Design review of the part built by this model. Coordinates are the model's own, in mm. Face numbers are marked on the shaded views. A direction names the side the tool comes from. Give positions to 0.01 mm unless a question says otherwise; leave off trailing zeros. Order: outer loops, then holes, each group sorted by start corner. A loop starts at its lowest first (then second) coordinate and runs counter-clockwise, first axis right, second up. Notation, with made-up numbers: M 76,-25 L 122,-25 A14 ccw 122,-20 Z; hole C -17.75,-0.75 d1. An arc over 180 degrees is marked long. Answer as a JSON object with one key per item and string values.
from build123d import *

# Parameters (mm, degrees)
F0_W     = 200
F0_H     = 164
F0_R     = 67
F0_H_2   = 12
F0_R_2   = 53
F1_DEPTH = 12
F2_W     = 12
F2_H     = 69
F2_H_2   = 12
F2_H_3   = 152
F2_W_2   = 6
F3_DEPTH = 276
F4_W     = 200
F4_H     = 257
F5_DEPTH = 12


with BuildPart() as f1:
    # F0 (on Front) → F1 (new body)
    with BuildSketch(Plane.XZ):
        with Locations((0, -46.5)):
            Rectangle(F0_W, F0_H)
        with Locations((0, -40.5)):
            Circle(F0_R, mode=Mode.SUBTRACT)
        Polygon((100, 128.5), (-100, 128.5), (-100, 47.5), (100, 47.5), (100, 67.5), (30, 67.5), (30, 108.5), (100, 108.5), align=None)
        with Locations((0, 41.5)):
            Rectangle(F0_W, F0_H_2)
        with Locations((0, -40.5)):
            Circle(F0_R)
        with Locations((0, -40.5)):
            Circle(F0_R_2, mode=Mode.SUBTRACT)
    extrude(amount=F1_DEPTH)

    # F2 (on face) → F3 (join)
    with BuildSketch(Plane(origin=(0, 0, 0), x_dir=(-1, 0, 0), z_dir=(0, 1, 0))):
        Polygon((100, 128.5), (-100, 128.5), (-100, 116.5), (88, 116.5), (100, 116.5), align=None)
        with Locations((94, 82)):
            Rectangle(F2_W, F2_H)
        with Locations((94, 41.5)):
            Rectangle(F2_W, F2_H_2)
        Polygon((88, 35.5), (88, 47.5), (-100, 47.5), (-100, 35.5), (-94, 35.5), align=None)
        with Locations((94, -40.5)):
            Rectangle(F2_W, F2_H_3)
        Polygon((100, -128.5), (100, -116.5), (88, -116.5), (-94, -116.5), (-100, -116.5), (-100, -128.5), align=None)
        with Locations((-97, -40.5)):
            Rectangle(F2_W_2, F2_H_3)
    extrude(amount=F3_DEPTH)

    # F4 (on face) → F5 (join)
    with BuildSketch(Plane(origin=(0, 276, 0), x_dir=(-1, 0, 0), z_dir=(0, 1, 0))):
        Rectangle(F4_W, F4_H)
    extrude(amount=F5_DEPTH)

    # F6: F1 across face


with BuildPart() as f1_1:
    add(f1.part)
    add(f1.part.mirror(Plane(origin=(100, 139.230769, -27.880342), x_dir=(0, 1, 0), z_dir=(1, 0, 0))))


solid = f1_1.part
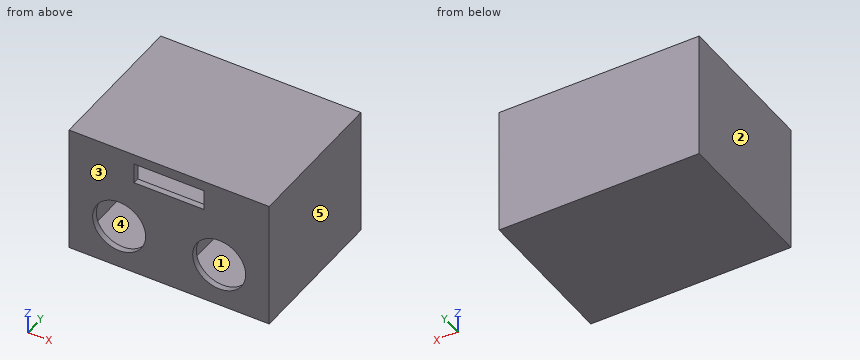
(1) Draft analysis for pull direction Y (two halves, no side actions). For the marked faces 3, 4 and 5, state which applies: +Y half, -Y half, draft (parallel to the pull), parting line (faces both ways), or undercut.
Checked values:
{"face 3": "-Y half", "face 4": "undercut", "face 5": "draft"}
(2) We need section C-C (z = -40.5). Write out the cut boundary in (x, y).
Checked values:
{"outline": "M -100,-12 L -53,-12 L -53,0 L -88,0 L -88,276 L 94,276 L 94,0 L 53,0 L 53,-12 L 147,-12 L 147,0 L 106,0 L 106,276 L 288,276 L 288,0 L 253,0 L 253,-12 L 300,-12 L 300,288 L -100,288 Z"}
(3) Tool access review of the marked faces 1 and 2: name each direction out of +Z, -Z, +X, -X, +Y, -Y from which nothing blocks a thin tool from reaching the whole face with its end or side.
Checked values:
{"face 1": "none", "face 2": "+Z, -Z, -X, +Y, -Y"}
(4) We need section A-A (x = 0). Write out the cut boundary in (y, z), plus the area to 3 significant figures.
Checked values:
{"outline": "M -12,-128.5 L 288,-128.5 L 288,128.5 L -12,128.5 L -12,12.5 L 0,12.5 L 0,35.5 L 276,35.5 L 276,-116.5 L 0,-116.5 L 0,-93.5 L -12,-93.5 Z; hole M 0,47.5 L 276,47.5 L 276,116.5 L 0,116.5 Z", "area": "14,800 mm^2"}
(5) We need section B-B (y = 245.5). Write out the cut boundary in (x, z).
Checked values:
{"outline": "M -100,-128.5 L 300,-128.5 L 300,128.5 L -100,128.5 Z; hole M -88,-116.5 L 94,-116.5 L 94,35.5 L -88,35.5 Z; hole M -88,47.5 L 288,47.5 L 288,116.5 L -88,116.5 Z; hole M 106,-116.5 L 288,-116.5 L 288,35.5 L 106,35.5 Z"}
(6) To check wall thickness, follow L1, parallel to Z at x = 247, y = 13; L2, parallel to X at y = 196, z = -97.5; L3, parallel to X at y = -9, z = -40. State the ranges of each line that lie inside material, in increasing order. Write a range as from..to.
Checked values:
{"L1": "z = -128.5..-116.5, 35.5..47.5, 116.5..128.5", "L2": "x = -100..-88, 94..106, 288..300", "L3": "x = -100..-53, 53..147, 253..300"}
(7) We need section D-D (x = 272). Write out the cut boundary in (y, z).
Checked values:
{"outline": "M -12,-128.5 L 288,-128.5 L 288,128.5 L -12,128.5 Z; hole M 0,-116.5 L 276,-116.5 L 276,35.5 L 0,35.5 Z; hole M 0,47.5 L 276,47.5 L 276,116.5 L 0,116.5 Z"}
